```python
from build123d import *

# Parameters (mm, degrees)
SKETCH1_W           = 39.878
SKETCH1_H           = 39.878
SKETCH1_W_2         = 35.052
SKETCH1_H_2         = 35.052
BOSS_EXTRUDE1_DEPTH = 300
SKETCH2_R           = 19.939
CUT_EXTRUDE1_DEPTH  = 300
SKETCH3_R           = 5
CUT_EXTRUDE2_DEPTH  = 95


with BuildPart() as part:
    # Sketch1 → Boss-Extrude1 (new body)
    with BuildSketch(Plane.XY):
        Rectangle(SKETCH1_W, SKETCH1_H)
        Rectangle(SKETCH1_W_2, SKETCH1_H_2, mode=Mode.SUBTRACT)
    extrude(amount=BOSS_EXTRUDE1_DEPTH)

    # Sketch2 → Cut-Extrude1 (cut)
    with BuildSketch(Plane(origin=(19.939, 0, 0), x_dir=(0, 0, -1), z_dir=(1, 0, 0))):
        with Locations((-300, 0)):
            Circle(SKETCH2_R)
        Circle(SKETCH2_R)
    extrude(amount=-CUT_EXTRUDE1_DEPTH, mode=Mode.SUBTRACT)

    # Sketch3 → Cut-Extrude2 (cut)
    with BuildSketch(Plane(origin=(0, 19.939, 0), x_dir=(1, 0, 0), z_dir=(0, 1, 0))):
        with Locations(Location((0, -198.315, 0), (0, 0, 270))):
            Circle(SKETCH3_R)
        with Locations(Location((0, -254.545, 0), (0, 0, 270))):
            Circle(SKETCH3_R)
        with Locations(Location((0, -101.685, 0), (0, 0, 270))):
            Circle(SKETCH3_R)
        with Locations(Location((0, -45.455, 0), (0, 0, 270))):
            Circle(SKETCH3_R)
    extrude(amount=-CUT_EXTRUDE2_DEPTH, mode=Mode.SUBTRACT)


solid = part.part
```
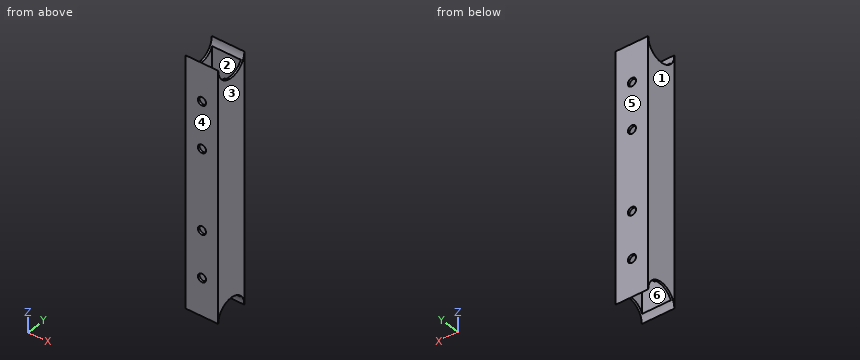
Source: CAD feature listing. Evaluate the final solid. Frame: model axes, mm. Face numbers are marked on the shaded views. A direction names the side the tool comes from. Round coordinates to 2 decimals unless told otherwise and drop trailing zeros. Loops run counter-clockwise (first coordinate to the right, second up) from the corner with the lowest first, then second, coordinate; pieces in that order, holes last. Notation, with made-up numbers: M 55,76.5 L 76,76.5 A18 ccw 76,111.5 Z; hole C 25.5,19 d6. An arc over 180 degrees is marked long. Use a Markdown table: item, result. Add a question column.
1. Reachability of the marked faces 1 and 2 from +Z, -Z, +X, -X, +Y, -Y: full face, straight path, thin tool, end or side. Return the list, or none.
2. Section query C-C on y = 0. Return the cut outline in (x, z), then the cut area to 3 significant figures.
3. Mould query, pull axis Y, two halves, no side actions, for the marked faces 3, 4, 5 and 6. Classes: pulls with the +Y half, pulls with the -Y half, needs draft (parallel to the pull), parting line crosses it, or undercut.
4. Section query A-A on x = -7.5. Return the cut outline in (y, z), then the cut area to 3 significant figures.
5. Contact query for flat-ended pins moving along their axis: P1, Ø9, axis at x = 0, z = 254.545, coming from the +Y side (3 decimals); P2, Ø8, axis at x = 15, y = -14, coming from the +Z side. Output: stop coordinate, or through.
6. Section query B-B on z = 70.5. Return the cut outline in (x, y), then the cut area to 3 significant figures.
7. Line query: line 1 (X direction, y = 5, z = 221); line 2 (Z direction, x = 4, y = 18) (3 decimals). Output: solid intervals per line, ascending.
Reported:
| question | item | result |
|---|---|---|
| 1 | face 1 | +Z, -Z, -X, +Y, -Y |
| 1 | face 2 | +Z, -Z |
| 2 | outline | M -19.94,19.94 L -17.53,19.94 L -17.53,280.06 L -19.94,280.06 Z; M 17.53,19.94 L 19.94,19.94 L 19.94,280.06 L 17.53,280.06 Z |
| 2 | area | 1,260 mm² |
| 3 | face 3 | needs draft |
| 3 | face 4 | pulls with the -Y half |
| 3 | face 5 | pulls with the +Y half |
| 3 | face 6 | undercut |
| 4 | outline | M -19.94,0 A19.94 cw -17.53,9.51 L -17.53,290.49 A19.94 cw -19.94,300 Z; M 17.53,9.51 A19.94 cw 19.94,0 L 19.94,300 A19.94 cw 17.53,290.49 Z |
| 4 | area | 1,390 mm² |
| 5 | P1 | passes through |
| 5 | P2 | stops at z = 291.42 |
| 6 | outline | M -19.94,-19.94 L 19.94,-19.94 L 19.94,19.94 L -19.94,19.94 Z; hole M -17.53,-17.53 L 17.53,-17.53 L 17.53,17.53 L -17.53,17.53 Z |
| 6 | area | 362 mm² |
| 7 | line 1 | x = -19.94 to -17.53, 17.53 to 19.94 |
| 7 | line 2 | z = 8.577 to 42.455, 48.455 to 98.685, 104.685 to 195.315, 201.315 to 251.545, 257.545 to 291.423 |
